Verification items for the finished model (mm, model axes). A direction names the side the tool comes from. Round coordinates to 2 decimals unless told otherwise and drop trailing zeros. Order: outer loops, then holes, each group sorted by start corner. A loop starts at its lowest first (then second) coordinate and runs counter-clockwise, first axis right, second up. Notation, with made-up numbers: (-20, 3.25) -> (26, 3.25) arc R33 cw to (26, 39.25) -> close; hole circle Ø6 at (67, 44.5). An arc over 180 degrees is marked (long way). Answer in a Markdown table with one row per item. Add a question column.
```python
from build123d import *

# Parameters (mm, degrees)
MODEL_R             = 11
MODEL_R_2           = 4
MODEL_R_3           = 1
MODEL_R_4           = 2.5
BOSS_EXTRUDE1_DEPTH = 12.4


with BuildPart() as part:
    # Model → Boss-Extrude1 (new body)
    with BuildSketch(Plane.XY):
        Polygon((-45, 0), (-50, 5), (-50, 50), (-40, 50), (-40, 62.4), (-10, 62.4), (-10, 50), (10, 50), (10, 62.4), (40, 62.4), (40, 50), (50, 50), (50, 5), (45, 0), align=None)
        with Locations(Location((0, 19.6, 0), (0, 0, 180))):
            Circle(MODEL_R, mode=Mode.SUBTRACT)
        with Locations(Location((-35, 19.6, 0), (0, 0, 180))):
            Circle(MODEL_R_2, mode=Mode.SUBTRACT)
        with Locations(Location((35, 19.6, 0), (0, 0, 180))):
            Circle(MODEL_R_2, mode=Mode.SUBTRACT)
        with Locations(Location((-35, 26.6, 0), (0, 0, 180))):
            Circle(MODEL_R_3, mode=Mode.SUBTRACT)
        with Locations(Location((-35, 12.6, 0), (0, 0, 180))):
            Circle(MODEL_R_3, mode=Mode.SUBTRACT)
        with Locations(Location((35, 12.6, 0), (0, 0, 180))):
            Circle(MODEL_R_3, mode=Mode.SUBTRACT)
        with Locations(Location((35, 26.6, 0), (0, 0, 180))):
            Circle(MODEL_R_3, mode=Mode.SUBTRACT)
        with Locations(Location((-18, 19.6, 0), (0, 0, 180))):
            Circle(MODEL_R_4, mode=Mode.SUBTRACT)
        with Locations(Location((18, 19.6, 0), (0, 0, 180))):
            Circle(MODEL_R_4, mode=Mode.SUBTRACT)
    extrude(amount=BOSS_EXTRUDE1_DEPTH)


solid = part.part
```
1) Cross-section at B-B, the plane y = 51. Record the boundary of the cut face in (x, z), and give its area (3 significant figures).
2) Cross-section at D-D, the plane z = 7.25. Give the number of separate pieces and of enclosed holes in the cut face, and give its area (3 significant figures).
3) Cross-section at A-A, the plane x = 0. Record the boundary of the cut face in (y, z), and give its area (3 significant figures).
4) Cross-section at C-C, the plane x = 35. Record the boundary of the cut face in (y, z), and give its area (3 significant figures).
5) Draft check along Y on faces 1 (the face through (-10, 56, 6)), 2 (the face through (1, 0, 6)), 3 (the face through (-34.87, 25.61, 6.11)). Enter one of: +Y half, -Y half, draft (parallel to the pull), parting line (faces both ways), or undercut.
6) Thickness scan on L1, parallel to Y at x = -35, z = 6.5; L2, parallel to X at y = 19.6, z = 8.5; L3, parallel to Y at x = -18, z = 7. Record the ranges inside material, lowest first. Write a range as [from, to].
7) Tool access check on faces 4 (the face through (-45, 50, 6)), 5 (the face through (0, 50, 6)), 6 (the face through (40, 56, 6)). Record the directions out of +Z, -Z, +X, -X, +Y, -Y that give a thin tool (end or side, any length) a straight path to the whole face; none if there is none.
8) Depth check by flat-ended pin: P1, Ø6, axis at y = 56, z = 4.5, coming from the -X side; P2, Ø3, axis at x = 46, z = 5, coming from the +Y side. Enter the tip coordinate at first touch or a pass-through.
Results below:
| question | item | result |
|---|---|---|
| 1 | outline | (-40, 0) -> (-10, 0) -> (-10, 12.4) -> (-40, 12.4) -> close; (10, 0) -> (40, 0) -> (40, 12.4) -> (10, 12.4) -> close |
| 1 | area | 744 mm² |
| 2 | separate pieces | 1 |
| 2 | enclosed holes | 9 |
| 2 | area | 5,190 mm² |
| 3 | outline | (0, 0) -> (8.6, 0) -> (8.6, 12.4) -> (0, 12.4) -> close; (30.6, 0) -> (50, 0) -> (50, 12.4) -> (30.6, 12.4) -> close |
| 3 | area | 347 mm² |
| 4 | outline | (0, 0) -> (11.6, 0) -> (11.6, 12.4) -> (0, 12.4) -> close; (13.6, 0) -> (15.6, 0) -> (15.6, 12.4) -> (13.6, 12.4) -> close; (23.6, 0) -> (25.6, 0) -> (25.6, 12.4) -> (23.6, 12.4) -> close; (27.6, 0) -> (62.4, 0) -> (62.4, 12.4) -> (27.6, 12.4) -> close |
| 4 | area | 625 mm² |
| 5 | face 1 | draft |
| 5 | face 2 | -Y half |
| 5 | face 3 | undercut |
| 6 | L1 | [0, 11.6], [13.6, 15.6], [23.6, 25.6], [27.6, 62.4] |
| 6 | L2 | [-50, -39], [-31, -20.5], [-15.5, -11], [11, 15.5], [20.5, 31], [39, 50] |
| 6 | L3 | [0, 17.1], [22.1, 62.4] |
| 7 | face 4 | +Z, -Z, -X, +Y |
| 7 | face 5 | +Z, -Z, +Y |
| 7 | face 6 | +Z, -Z, +X, +Y |
| 8 | P1 | x = -40 |
| 8 | P2 | y = 50 |
